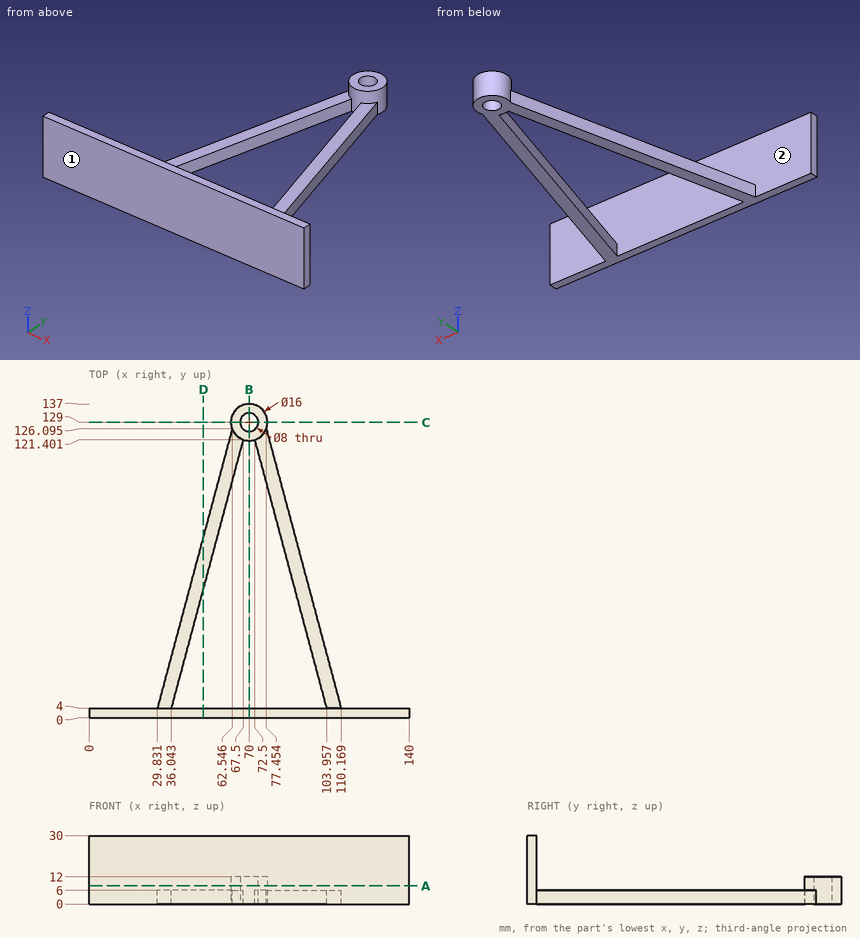
Can you work these out from the drawing? Everything is in mm from the part's minimum corner. Round coordinates to 2 decimals unless told otherwise and drop trailing zeros. Order: outer loops, then holes, each group sorted by start corner. A loop starts at its lowest first (then second) coordinate and runs counter-clockwise, first axis right, second up.
(1) If we section it at C-C (y = 129): Please give me the cut outline in (x, z).
Results are:
outline: (62, 0) - (66, 0) - (66, 12) - (62, 12) - close; (74, 0) - (78, 0) - (78, 12) - (74, 12) - close
(2) If we section it at D-D (x = 50): Please give me the cut outline in (y, z).
Results are:
outline: (0, 0) - (4, 0) - (4, 30) - (0, 30) - close; (56.09, 0) - (79.27, 0) - (79.27, 6) - (56.09, 6) - close
(3) If I drill on L1, parallel to Y at x = 70, z = 6.75; L2, parallel to Y at x = 66.5, z = 11.5 (1 decimal); L3, parallel to Y at x = 120, z = 7.5, over which ranges is the centre line in solid material (lowest first)?
Results are:
L1: y = 0 to 4, 121 to 125, 133 to 137
L2: y = 0 to 4, 121.8 to 127.1, 130.9 to 136.2
L3: y = 0 to 4
(4) If we section it at B-B (x = 70): Please give me the cut outline in (y, z), plus the area to 3 significant figures.
Results are:
outline: (0, 0) - (4, 0) - (4, 30) - (0, 30) - close; (121, 0) - (125, 0) - (125, 12) - (121, 12) - close; (133, 0) - (137, 0) - (137, 12) - (133, 12) - close
area: 216 mm2
(5) We'd pull the mould along X, two halves only. Please class the marked faces 1 and 2: +X half, -X half, draft (parallel to the pull), parting line (faces both ways), or undercut.
Results are:
face 1: draft
face 2: undercut
(6) If we section it at A-A (z = 8): Please give me the cut outline in (x, y).
Results are:
outline: (0, 0) - (140, 0) - (140, 4) - (0, 4) - close; circle Ø16 at (70, 129); hole circle Ø8 at (70, 129)
(7) I'm going to push flat-ended pins straight in: pin 1 (8 mm diameter, centred on y = 75.5, z = 12, fed in from +X); pin 2 (17.5 mm diameter, centred on x = 70.5, y = 128, fed in from +Z); pin 3 (19 mm diameter, centred on x = 84, y = 82.5, fed in from +Z); pin 4 (8 mm diameter, centred on y = 121, z = 6.5, fed in from +X). Where does each tip first touch, or does it pass through?
Results are:
pin 1: passes through
pin 2: stops at z = 12
pin 3: stops at z = 6
pin 4: stops at x = 79.88
